Here's the drawing with two shaded views (mm, measured from the low corner). I have some questions. Coordinates: 2 decimals unless noted, no trailing zeros. Loops run counter-clockwise (first coordinate to the right, second up) from the corner with the lowest first, then second, coordinate; pieces in that order, holes last. Notation, with made-up numbers: (88, 46) -> (131, 46) arc R28 ccw to (131, 83) -> close; hole circle Ø5 at (82, 51.5). An arc over 180 degrees is marked (long way). Answer as a JSON object with one key per item and string values. Group by question number.
Q1. I need wall thicknesses on line 1 (Z direction, x = 28.5, y = 24); line 2 (Y direction, x = 18, z = 80); line 3 (Z direction, x = 28, y = 19.5). Which ranges of each line are inside material? Lowest first, please.
Q2. I want a section at A-A on y = 25. Write out the boundary of the cut face in (x, z), then the cut area to 3 significant figures.
Q3. I want a section at B-B on z = 345. Write out the boundary of the cut face in (x, y), then the cut area to 3 significant figures.
Q4. I want a section at C-C on x = 24.5. Write out the boundary of the cut face in (y, z), then the cut area to 3 significant figures.
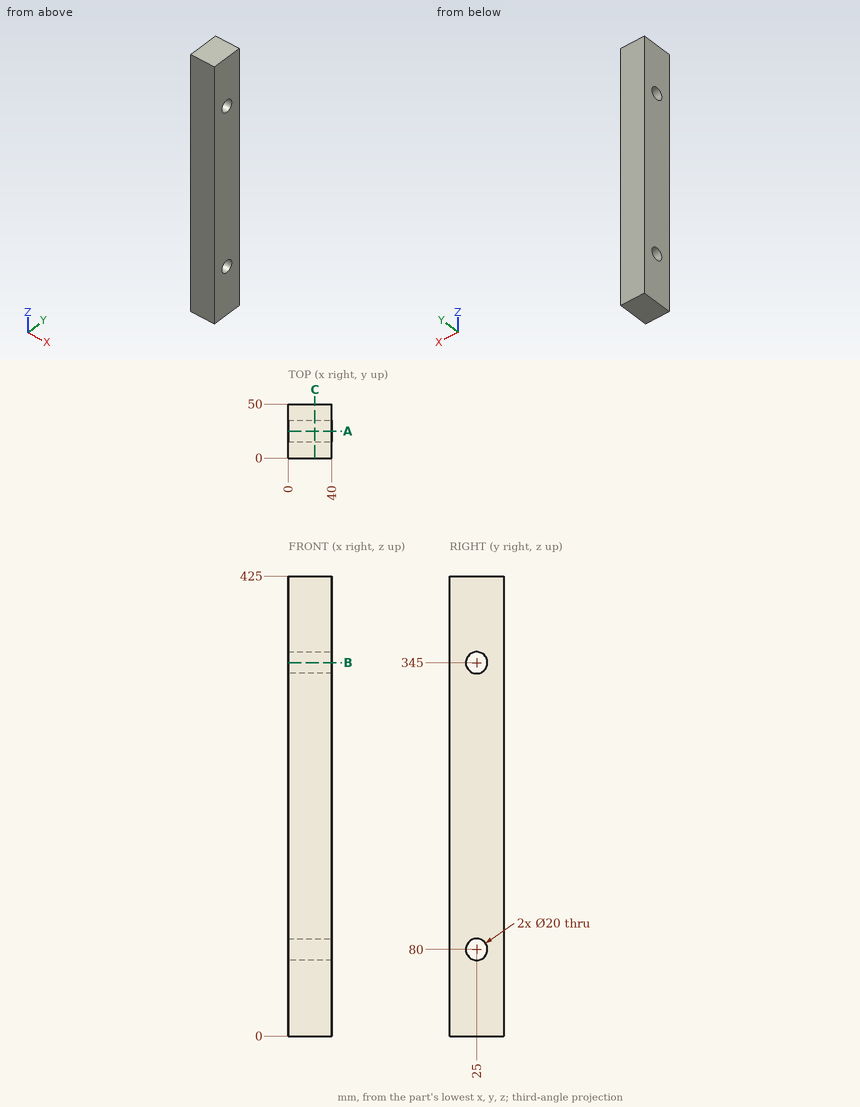
Result set:
{
 "1": {"line 1": "z = 0 to 70.05, 89.95 to 335.05, 354.95 to 425", "line 2": "y = 0 to 15, 35 to 50", "line 3": "z = 0 to 71.65, 88.35 to 336.65, 353.35 to 425"},
 "2": {"outline": "(0, 0) -> (40, 0) -> (40, 70) -> (0, 70) -> close; (0, 90) -> (40, 90) -> (40, 335) -> (0, 335) -> close; (0, 355) -> (40, 355) -> (40, 425) -> (0, 425) -> close", "area": "15,400 mm²"},
 "3": {"outline": "(0, 0) -> (40, 0) -> (40, 15) -> (0, 15) -> close; (0, 35) -> (40, 35) -> (40, 50) -> (0, 50) -> close", "area": "1,200 mm²"},
 "4": {"outline": "(0, 0) -> (50, 0) -> (50, 425) -> (0, 425) -> close; hole circle Ø20 at (25, 80); hole circle Ø20 at (25, 345)", "area": "20,600 mm²"}
}
